Autodesk Inventor part; units mm, degrees
ref_plane "YZ Plane" through (0, 0, 0) normal (1, 0, 0) x (0, 1, 0)
ref_plane "XZ Plane" through (0, 0, 0) normal (0, 1, 0) x (-1, 0, 0)
ref_plane "XY Plane" through (0, 0, 0) normal (0, 0, 1) x (1, 0, 0)
sketch "Sketch1" plane through (0, 0, 0) normal (0, 0, 1) x (1, 0, 0)
  circle A0 centre (100.5809, -7) radius 2.5
  circle A1 centre (25.1452, -7) radius 2.5
  line L0 (0, 0) -> (125.7261, 0)
  line L1 (13.1452, 0) -> (112.5809, 0)
  line L2 (112.5809, 0) -> (112.5809, -14)
  line L3 (112.5809, -14) -> (13.1452, -14)
  line L4 (13.1452, -14) -> (13.1452, 0)
  dimension "d0" = 5
  dimension "d1" = 100.5809
  dimension "d2" = 125.7261
  dimension "d3" = 25.1452
  dimension "d4" = 7
  dimension "d5" = 7
  dimension "d8" = 12
  dimension "d9" = 12
  dimension "d10" = 7
  dimension "d23" = 99.4357
extrude "Extrusion1" add sketch "Sketch1" along normal blind 74
ref_plane "Work Plane1" through (0, 0, 64) normal (0, 0, 1) x (1, 0, 0)
sketch "Sketch2" plane through (0, 0, 64) normal (0, 0, 1) x (1, 0, 0)
  circle A0 centre (25.1452, -7) radius 2.5
  circle A1 centre (100.5809, -7) radius 2.5
  line L0 (25.1452, -12.1962) -> (20.6452, -9.5981)
  line L1 (20.6452, -9.5981) -> (20.6452, 0)
  line L2 (29.6452, 0) -> (29.6452, -9.5981)
  line L3 (29.6452, -9.5981) -> (25.1452, -12.1962)
  line L4 (100.5809, -12.1962) -> (96.0809, -9.5981)
  line L5 (96.0809, -9.5981) -> (96.0809, 0)
  line L6 (105.0809, 0) -> (105.0809, -9.5981)
  line L7 (105.0809, -9.5981) -> (100.5809, -12.1962)
  line L8 (13.1452, 0) -> (112.5809, 0)
  line L9 (20.6452, 0) -> (29.6452, 0)
  line L10 (96.0809, 0) -> (105.0809, 0)
  point P0 (0, 0)
  dimension "d27" = 9
  dimension "d28" = 9
extrude "Extrusion2" cut sketch "Sketch2" against normal blind 4 contours A0 | L8 L6 L7 L4 L5 | L0 L1 L8 L2 L3
sketch "Sketch3" plane through (0, 0, 0) normal (0, 0, -1) x (-1, 0, 0)
  circle A0 centre (-135.3631, -7) radius 4.5
  circle A1 centre (9.6369, -7) radius 4.5
  arc A2 (-128.6549, -1) -> (-128.6549, -13) centre (-135.3631, -7) ccw
  arc A3 (2.9287, -13) -> (2.9287, -1) centre (9.6369, -7) ccw
  line L0 (-134.0226, -7) -> (-135.886, -7) construction
  line L1 (-135.886, -7) -> (31.817, -7) construction
  line L2 (-112.5809, -14) -> (-13.1452, -14) construction
  line L3 (-13.1452, 0) -> (-112.5809, 0) construction
  line L4 (-128.6549, -1) -> (2.9287, -1)
  line L5 (2.9287, -13) -> (-128.6549, -13)
  circle A4 centre (-100.5809, -7) radius 2.5
  circle A5 centre (-25.1452, -7) radius 2.5
  point P0 (0, 0)
  dimension "d32" = 145
  dimension "d33" = 9
  dimension "d34" = 18
  dimension "d35" = 14
  dimension "d36" = 7
  dimension "d40" = 12
  dimension "d42" = 75.4357
  dimension "d43" = 34.7822
extrude "Extrusion3" add sketch "Sketch3" along normal blind 10
equation "\"d1\" = 0.8 * d2"
equation "\"d3\" = 0.2 * d2"
equation "\"d5\" = d4"
equation "\"d9\" = d8"
equation "\"d28\" = d27"
equation "\"d43\" = -0.5 * d42 + 0.5 * d32"
properties part number "license_mount"
The listing builds one solid part. Answer for the finished solid, in the listing's coordinates (mm). A direction names the side the tool comes from. Give positions to 0.01 mm unless a question says otherwise; leave off trailing zeros. Loops run counter-clockwise (first coordinate to the right, second up) from the corner with the lowest first, then second, coordinate; pieces in that order, holes last.
Item 1: Find the intervals of material crossed by line 1 along X through (y, z) = (-7, 45); line 2 along Z through (x, y) = (97.5, -9.75); line 3 along X through (y, z) = (-3.25, 34.5), in increasing order.
Derived:
line 1: x = 13.15 to 22.65, 27.65 to 98.08, 103.08 to 112.58
line 2: z = -10 to 60, 64 to 74
line 3: x = 13.15 to 112.58
Item 2: Determine the mould class of faces 4 (the flat face through (64, -7, -10)), 5 (the flat face through (-3, -7, 0)), 6 (the flat face through (101, -3, 64)), 7 (the cylindrical face through (144.36, -7.3, -4.93)) for opening direction Z: +Z half, -Z half, draft (parallel to the pull), parting line (faces both ways), or undercut.
Derived:
face 4: -Z half
face 5: +Z half
face 6: undercut
face 7: draft
Item 3: Each of these flat-tipped pins is pushed along its axis until it touches: pin 1 Ø8 at (x, z) = (95, -5) entering from -Y; pin 2 Ø0.5 at (x, y) = (67, -0.5) entering from -Z; pin 3 Ø4 at (x, y) = (0.5, -7) entering from +Z. Where does it stop, or does it pass through?
Derived:
pin 1: stops at y = -13
pin 2: stops at z = 0
pin 3: stops at z = 0
Item 4: A cutting plane is placed at A-A (z = -2). Give the vertices of the cut face in (x, y).
Derived:
outline: (-2.93, -13) - (128.65, -13) arc R9 ccw (long way) to (128.65, -1) - (-2.93, -1) arc R9 ccw (long way) to start; hole circle Ø9 at (-9.64, -7); hole circle Ø5 at (25.15, -7); hole circle Ø5 at (100.58, -7); hole circle Ø9 at (135.36, -7)
Item 5: A cutting plane is placed at C-C (z = 42.5). Give the vertices of the cut face in (x, y).
Derived:
outline: (13.15, -14) - (112.58, -14) - (112.58, 0) - (13.15, 0) - close; hole circle Ø5 at (25.15, -7); hole circle Ø5 at (100.58, -7)
Item 6: A cutting plane is placed at D-D (y = -7). Give the number of separate pieces and of enclosed holes in the cut face, then the cut area to 3 significant figures.
Derived:
separate pieces: 5
enclosed holes: 0
area: 7,940 mm2
Item 7: A cutting plane is placed at B-B (x = 85). Give the vertices of the cut face in (y, z), then the cut area to 3 significant figures.
Derived:
outline: (-14, 0) - (-13, 0) - (-13, -10) - (-1, -10) - (-1, 0) - (0, 0) - (0, 74) - (-14, 74) - close
area: 1,160 mm2
Item 8: A tool of negligible diameter and unlimited length cuts with its end or side. For faces 1 (the flat face through (129, -7, 0)), 2 (the flat face through (102.86, -10.88, 62.03)), 3 (the flat face through (62, -13, -5)), from which of +Z, -Z, +X, -X, +Y, -Y can it reach the whole face along a straight path? Write none if from no direction.
Derived:
face 1: +Z, +X, +Y, -Y
face 2: +Y
face 3: -Z, -Y
